from build123d import *

# Parameters (mm, degrees)
F0_W          = 76.5
F0_H          = 35.5
F1_DEPTH      = 4
F2_W          = 72.5
F2_H          = 31.5
F3_DEPTH      = 1
F5_R          = 6
F7_DEPTH      = 1
F6_R          = 6
F8_DEPTH      = 1
F13_DEPTH     = 3
F14_R         = 2.5
F15_T1_DEPTH  = 11.5
F15_T4_ANGLE  = 90
F15_T6_ANGLE  = 90
F15_T8_ANGLE  = 90
F15_T10_ANGLE = 90


# Not quite as in the source:
# - a fillet or chamfer that OpenCascade refuses, or shapes differently, is made with other operations: its cross-section is extruded or revolved along the edge and cut away or added


with BuildPart() as f1:
    # F0 (on Front) → F1 (new body)
    with BuildSketch(Plane.XZ):
        Rectangle(F0_W, F0_H)
    extrude(amount=F1_DEPTH)

    # F2 (on face) → F3 (cut)
    with BuildSketch(Plane.XZ.offset(4)):
        Rectangle(F2_W, F2_H)
    extrude(amount=-F3_DEPTH, mode=Mode.SUBTRACT)

    # F5 (on face) → F7 (join)
    with BuildSketch(Plane.XZ.offset(3)):
        with Locations((0, -2.25)):
            Circle(F5_R)
    extrude(amount=F7_DEPTH)

    # F6 (on face) → F8 (join)
    with BuildSketch(Plane.XZ.offset(3)):
        with Locations((19.25, -2.25)):
            Circle(F6_R)
        with Locations((-19.25, -2.25)):
            Circle(F6_R)
    extrude(amount=F8_DEPTH)

    # F9: chamfer of 2 x 3.5 on 3 edges, made by hand


with BuildPart() as f9_tool2:
    # F9_s3 → F9_t4 (revolve)
    with BuildSketch(Plane.XY.offset(-2.25)):
        Polygon((6, -0.5), (4, -4), (6, -4), align=None)
    revolve(axis=Axis((0, -4, -2.25), (0, -1, 0)))

    split(bisect_by=Plane.XZ.offset(3), keep=Keep.TOP)


with BuildPart() as f1_1:
    add(f1.part)

    # F9_t1: cut F9_tool2
    add(f9_tool2.part, mode=Mode.SUBTRACT)


with BuildPart() as f9_tool7:
    # F9_s8 → F9_t9 (revolve)
    with BuildSketch(Plane.XY.offset(-2.25)):
        Polygon((-13.25, -0.5), (-15.25, -4), (-13.25, -4), align=None)
    revolve(axis=Axis((-19.25, -4, -2.25), (0, -1, 0)))

    split(bisect_by=Plane.XZ.offset(3), keep=Keep.TOP)


with BuildPart() as f1_2:
    add(f1_1.part)

    # F9_t6: cut F9_tool7
    add(f9_tool7.part, mode=Mode.SUBTRACT)


with BuildPart() as f9_tool12:
    # F9_s13 → F9_t14 (revolve)
    with BuildSketch(Plane.XY.offset(-2.25)):
        Polygon((25.25, -0.5), (23.25, -4), (25.25, -4), align=None)
    revolve(axis=Axis((19.25, -4, -2.25), (0, -1, 0)))

    split(bisect_by=Plane.XZ.offset(3), keep=Keep.TOP)


with BuildPart() as f1_3:
    add(f1_2.part)

    # F9_t11: cut F9_tool12
    add(f9_tool12.part, mode=Mode.SUBTRACT)

    # F10 (on face) + F12 (on face) + F11 (on face) → F13 (cut)
    with BuildSketch(Plane.XZ.offset(4)):
        Polygon((-1.464609527, 0.2376197995), (-2.8866467048, -2.2745791573), (-1.4220371778, -4.7621989567), (1.464609527, -4.7376197995), (2.8866467048, -2.2254208427), (1.4220371778, 0.2621989567), align=None)
    with BuildSketch(Plane.XZ.offset(4)):
        Polygon((-17.806624327, 0.25), (-20.693375673, 0.25), (-22.1367513459, -2.25), (-20.693375673, -4.75), (-17.806624327, -4.75), (-16.3632486541, -2.25), align=None)
    with BuildSketch(Plane.XZ.offset(4)):
        Polygon((20.693375673, 0.25), (17.806624327, 0.25), (16.3632486541, -2.25), (17.806624327, -4.75), (20.693375673, -4.75), (22.1367513459, -2.25), align=None)
    extrude(amount=-F13_DEPTH, mode=Mode.SUBTRACT)

    # F14
    f14_edges = [f1_3.edges().sort_by_distance(p)[0] for p in [
        (0, 0, 17.75),
        (38.25, 0, 0),
        (0, 0, -17.75),
        (-38.25, 0, 0),
    ]]
    fillet(f14_edges, radius=F14_R)

    # F15: fillet of radius 3 on 8 edges, made by hand

    # F15_s2 → F15_t1 (cut)
    with BuildSketch(Plane.XZ):
        with BuildLine():
            ThreePointArc((35.25, 17.75), (37.3713203436, 16.8713203436), (38.25, 14.75))
            Line((38.25, 14.75), (38.25, 17.75))
            Line((38.25, 17.75), (35.25, 17.75))
        make_face()
        with BuildLine():
            ThreePointArc((38.25, -14.75), (37.3713203436, -16.8713203436), (35.25, -17.75))
            Line((35.25, -17.75), (38.25, -17.75))
            Line((38.25, -17.75), (38.25, -14.75))
        make_face()
        with BuildLine():
            ThreePointArc((-35.25, 17.75), (-37.3713203436, 16.8713203436), (-38.25, 14.75))
            Line((-38.25, 14.75), (-38.25, 17.75))
            Line((-38.25, 17.75), (-35.25, 17.75))
        make_face()
        with BuildLine():
            ThreePointArc((-38.25, -14.75), (-37.3713203436, -16.8713203436), (-35.25, -17.75))
            Line((-35.25, -17.75), (-38.25, -17.75))
            Line((-38.25, -17.75), (-38.25, -14.75))
        make_face()
    extrude(amount=F15_T1_DEPTH, mode=Mode.SUBTRACT)

    # F15_s3 → F15_t4 (revolve, cut)
    with BuildSketch(Plane.YZ.offset(35.25)):
        with BuildLine():
            ThreePointArc((0, 15.25), (-0.732233047, 17.017766953), (-2.5, 17.75))
            Line((-2.5, 17.75), (0, 17.75))
            Line((0, 17.75), (0, 15.25))
        make_face()
    revolve(axis=Axis((35.25, 0, 14.75), (0, 1, 0)), revolution_arc=F15_T4_ANGLE, mode=Mode.SUBTRACT)

    # F15_s5 → F15_t6 (revolve, cut)
    with BuildSketch(Plane.XY.offset(-14.75)):
        with BuildLine():
            ThreePointArc((35.75, 0), (37.517766953, -0.732233047), (38.25, -2.5))
            Line((38.25, -2.5), (38.25, 0))
            Line((38.25, 0), (35.75, 0))
        make_face()
    revolve(axis=Axis((35.25, 0, -14.75), (0, 1, 0)), revolution_arc=F15_T6_ANGLE, mode=Mode.SUBTRACT)

    # F15_s7 → F15_t8 (revolve, cut)
    with BuildSketch(Plane.XY.offset(14.75)):
        with BuildLine():
            ThreePointArc((-35.75, 0), (-37.517766953, -0.732233047), (-38.25, -2.5))
            Line((-38.25, -2.5), (-38.25, 0))
            Line((-38.25, 0), (-35.75, 0))
        make_face()
    revolve(axis=Axis((-35.25, 0, 14.75), (0, 1, 0)), revolution_arc=F15_T8_ANGLE, mode=Mode.SUBTRACT)

    # F15_s9 → F15_t10 (revolve, cut)
    with BuildSketch(Plane.YZ.offset(-35.25)):
        with BuildLine():
            ThreePointArc((0, -15.25), (-0.732233047, -17.017766953), (-2.5, -17.75))
            Line((-2.5, -17.75), (0, -17.75))
            Line((0, -17.75), (0, -15.25))
        make_face()
    revolve(axis=Axis((-35.25, 0, -14.75), (0, 1, 0)), revolution_arc=F15_T10_ANGLE, mode=Mode.SUBTRACT)


solid = f1_3.part
Check sheet for the modelled part. Datum: model origin and axes. Units: mm. A direction names the side the tool comes from. Round coordinates to 2 decimals unless told otherwise and drop trailing zeros. Loops run counter-clockwise (first coordinate to the right, second up) from the corner with the lowest first, then second, coordinate; pieces in that order, holes last.
1. Gauge pin test, flat ends, axial feed: pin 1 Ø1 at (y, z) = (-1.5, -5) entering from +X; pin 2 Ø5.5 at (x, z) = (-1.5, -2) entering from -Y; pin 3 Ø1 at (x, y) = (-23.5, -1.5) entering from +Z; pin 4 Ø1.5 at (x, z) = (20, -2) entering from -Y. Record the tip position at first contact, or that the pin passes through.
2. Sectioned sample at C-C on x = -30. Record the boundary of the cut face in (y, z), and give its area (3 significant figures).
3. Scan lines: probe 1 along X at (y, z) = (-2.45, -3); probe 2 along X at (y, z) = (-2.8, 15); probe 3 along Y at (x, z) = (2, -3). Record each from-to range of solid material in increasing order.
4. Mould release check, pull along X, two halves, no side actions. Record for faces 3 (the flat face through (-21.425, -2.521, -3.482)), 4 (the cylindrical face through (37.39, -3.24, -16.85)), 5 (the flat face through (0, -4, 16)): released by +X, released by -X, zero draft, split by the parting line, or undercut.
5. Sectioned sample at A-A on x = -19.25. Record the boundary of the cut face in (y, z).
6. Set-up check for faces 1 (the flat face through (2.166, -2.521, -3.499)), 2 (the flat face through (0, -4, -5)): record each of +Z, -Z, +X, -X, +Y, -Y from which the full face is reachable in a straight line by a thin tool's end or side.
7. Sectioned sample at B-B on z = 13. Record the boundary of the cut face in (x, y), and give its area (3 significant figures).
Recorded:
1. pin 1: stops at x = 38.2
1. pin 2: stops at y = -4
1. pin 3: stops at z = 17.7
1. pin 4: stops at y = -1
2. outline: (-4, -17.75) - (-2.5, -17.75) arc R2.5 ccw to (0, -15.25) - (0, 15.25) arc R2.5 ccw to (-2.5, 17.75) - (-4, 17.75) - (-4, 15.75) - (-3, 15.75) - (-3, -15.75) - (-4, -15.75) - close
2. area: 108 mm2
3. probe 1: x = -38.25 to -21.7, -16.8 to -2.46, 2.45 to 16.8, 21.7 to 38.25
3. probe 2: x = -38.24 to 38.24
3. probe 3: y = -1 to 0
4. face 3: undercut
4. face 4: released by +X
4. face 5: zero draft
5. outline: (-4, -17.75) - (-2.5, -17.75) arc R2.5 ccw to (0, -15.25) - (0, 15.25) arc R2.5 ccw to (-2.5, 17.75) - (-4, 17.75) - (-4, 15.75) - (-3, 15.75) - (-3, 2.32) - (-4, 1.75) - (-4, 0.25) - (-1, 0.25) - (-1, -4.75) - (-4, -4.75) - (-4, -6.25) - (-3, -6.82) - (-3, -15.75) - (-4, -15.75) - close
6. face 1: -Y
6. face 2: +Z, -Z, +X, -X, -Y
7. outline: (-38.25, -4) - (-36.25, -4) - (-36.25, -3) - (36.25, -3) - (36.25, -4) - (38.25, -4) - (38.25, -2.5) arc R2.5 ccw to (35.75, 0) - (-35.75, 0) arc R2.5 ccw to (-38.25, -2.5) - close
7. area: 231 mm2
